CAD build for the part. Positions are in the model's coordinates, mm. Give positions to 0.01 mm unless a question says otherwise; leave off trailing zeros. Loops run counter-clockwise (first coordinate to the right, second up) from the corner with the lowest first, then second, coordinate; pieces in that order, holes last. Notation, with made-up numbers: M 50.5,-33 L 55.5,-33 A15 cw 55.5,-20 Z; hole C 22.25,88.5 d9. An arc over 180 degrees is marked long. Answer as CSV lines item,"result".
Autodesk Inventor part; units mm, degrees
ref_plane "YZ Plane" through (0, 0, 0) normal (1, 0, 0) x (0, 1, 0)
ref_plane "XZ Plane" through (0, 0, 0) normal (0, 1, 0) x (-1, 0, 0)
ref_plane "XY Plane" through (0, 0, 0) normal (0, 0, 1) x (1, 0, 0)
sketch "Sketch2" plane through (0, 0, 0) normal (0, 1, 0) x (-1, 0, 0)
  circle A0 centre (0, 0) radius 7.5
  circle A1 centre (0, 0) radius 6.5
  dimension "d91" = 15
  dimension "d92" = 13
extrude "Extrusion5" add sketch "Sketch2" along normal blind 500
sketch "Sketch3" plane through (0, 0, 0) normal (0, 0, 1) x (1, 0, 0)
  line L0 (0, 0) -> (0, 6)
  circle A0 centre (0, 6) radius 1.5
  line L1 (7.5, 500) -> (-7.5, 500)
  line L2 (0, 500) -> (0, 485)
  circle A1 centre (0, 485) radius 1.5
  dimension "d95" = 6
  dimension "d96" = 3
  dimension "d101" = 15
  dimension "d102" = 3
extrude "Extrusion6" cut sketch "Sketch3" along normal blind 20 and the other way blind 10
properties part number "airfoil"
1) Band-saw the part on B-B on y = 309.5. Give the cut face in (x, z), and give its area (3 significant figures).
Answer below:
outline,"C 0,0 d15; hole C 0,0 d13"
area,"44.0 mm^2"
2) Band-saw the part on A-A on z = 0. Give the cut face in (x, y).
Answer below:
outline,"M -7.5,0 L -6.5,0 L -6.5,500 L -7.5,500 Z; M 6.5,0 L 7.5,0 L 7.5,500 L 6.5,500 Z"
3) Flat gauge pins, fed straight in: pin 1 (4 mm diameter, centred on x = -4, z = 1.5, fed in from +Y); pin 2 (6 mm diameter, centred on x = 0.5, y = 103, fed in from -Z); pin 3 (3 mm diameter, centred on x = 5.5, y = 398, fed in from +Z); pin 4 (3 mm diameter, centred on x = 2.5, y = 169.5, fed in from -Z). Where does each tip first touch, or does it go through?
Answer below:
pin 1,"passes through"
pin 2,"stops at z = -7.5"
pin 3,"stops at z = 6.34"
pin 4,"stops at z = -7.43"
4) Mould opens along X. For faces 1 (the face through (5.158, 246.5, 3.955)), 2 (the face through (6, 0, 3)), 3 (the face through (7.493, 246.5, -0.33)) say: +X half, -X half, draft (parallel to the pull), parting line (faces both ways), or undercut.
Answer below:
face 1,"undercut"
face 2,"draft"
face 3,"parting line"
5) Drill centre lines: line 1 (Y direction, x = 0, z = 7.1); line 2 (Z direction, x = 0.5, y = 98.5); line 3 (Y direction, x = 1, z = 7.25). Where is each one in solid material? Low to high. Write a range as from..to.
Answer below:
line 1,"y = 0..4.5, 7.5..483.5, 486.5..500"
line 2,"z = -7.48..-6.48, 6.48..7.48"
line 3,"y = 0..4.88, 7.12..483.88, 486.12..500"
